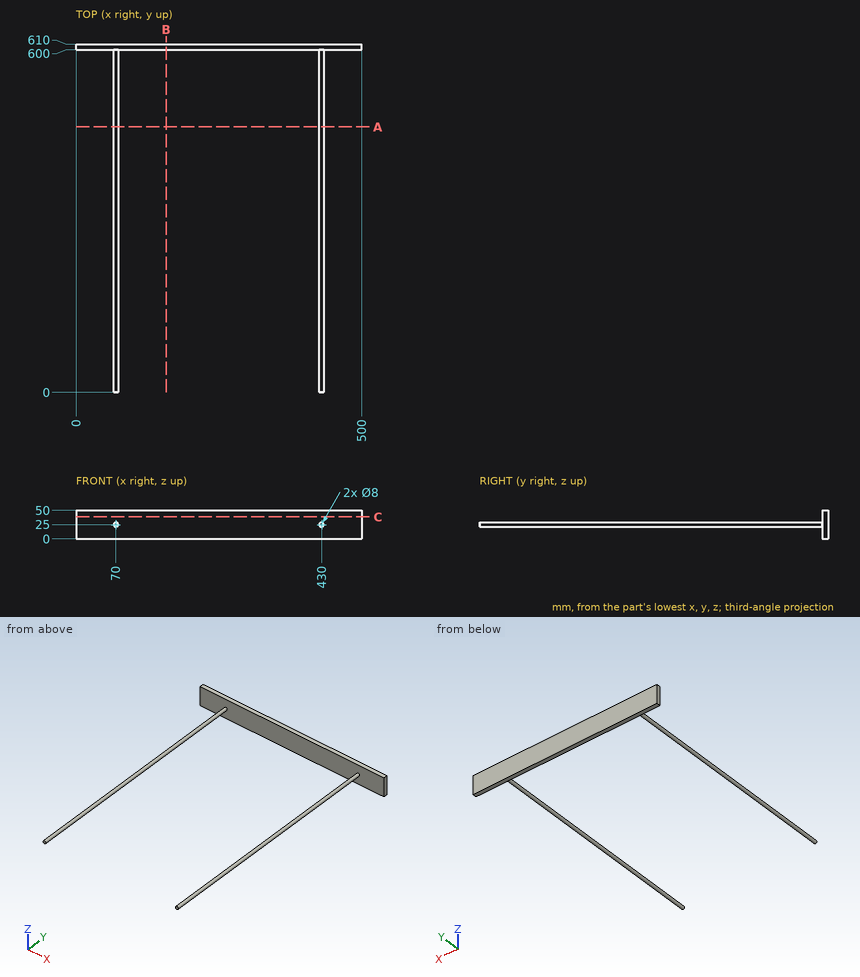
Verification items for this drawing (mm, ordinates from the low corner). Coordinates: 2 decimals unless noted, no trailing zeros. Order: outer loops, then holes, each group sorted by start corner. A loop starts at its lowest first (then second) coordinate and runs counter-clockwise, first axis right, second up. Notation, with made-up numbers: M 1,77 L 21,77 A4 ccw 21,82 Z; hole C 50,3.25 d2. An arc over 180 degrees is marked long. Use CSV: the item, a comma, the result in double quotes.
Item 1: Cross-section at B-B on x = 158. Record the cut outline in (y, z), then the cut area to 3 significant figures.
Returned:
outline,"M 600,0 L 610,0 L 610,50 L 600,50 Z"
area,"500 mm2"
Item 2: Cross-section at A-A on y = 465. Record the cut outline in (x, z).
Returned:
outline,"C 70,25 d8; C 430,25 d8"
Item 3: Thickness scan on line 1 along Y through (x, z) = (272, 37); line 2 along X through (y, z) = (409, 22.5); line 3 along X through (y, z) = (578.5, 23.5). Record the ranges inside material, lowest first.
Returned:
line 1,"y = 600 to 610"
line 2,"x = 66.88 to 73.12, 426.88 to 433.12"
line 3,"x = 66.29 to 73.71, 426.29 to 433.71"
Item 4: Cross-section at C-C on z = 38.5. Record the cut outline in (x, y).
Returned:
outline,"M 0,600 L 500,600 L 500,610 L 0,610 Z"
Item 5: Gauge pin test, flat ends, axial feed: pin 1 Ø12 at (x, z) = (278.5, 23.5) entering from -Y; pin 2 Ø4 at (y, z) = (437.5, 20) entering from -X. Record the tip position at first contact, or that the pin passes through.
Returned:
pin 1,"stops at y = 600"
pin 2,"stops at x = 67.35"
